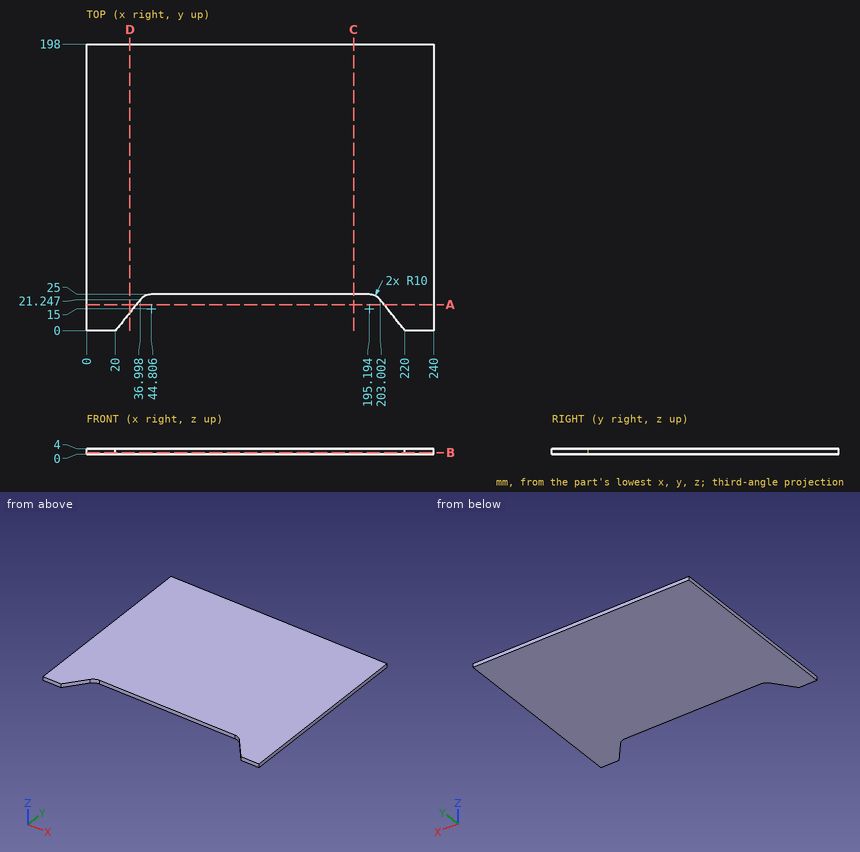
Part print with two shaded views. Sizes in mm from the minimum x, y, z corner. Round coordinates to 2 decimals unless told otherwise and drop trailing zeros. Order: outer loops, then holes, each group sorted by start corner. A loop starts at its lowest first (then second) coordinate and runs counter-clockwise, first axis right, second up. Notation, with made-up numbers: M 0.25,-0.75 L 26.25,-0.75 A16 cw 26.25,26.25 Z; hole C 84,57 d6. An arc over 180 degrees is marked long. Answer in a Markdown table with one row per item. Add a question column.
Q1. Wall check: L1, parallel to Y at x = 81.5, z = 0.35; L2, parallel to X at y = 15.5, z = 3.75; L3, parallel to Y at x = 37, z = 1.8. Give the ranges that are in metal, low to high. Write a range as from..to.
Q2. Pin check, flat tip, straight feed: pin 1 (1 mm diameter, centred on x = 51.5, z = 2, fed in from -Y). Stop position of the tip, or through.
Q3. Cut at D-D on x = 30. Give the cut face in (y, z).
Q4. Cut at C-C on x = 184.5. Give the cut face in (y, z).
Q5. Cut at A-A on y = 18. Give the cut face in (x, z).
Q6. Cut at B-B on z = 1.25. Give the cut face in (x, y), and give its area (3 significant figures).
Established:
| question | item | result |
|---|---|---|
| 1 | L1 | y = 25..198 |
| 1 | L2 | x = 0..32.4, 207.6..240 |
| 1 | L3 | y = 21.25..198 |
| 2 | pin 1 | stops at y = 25 |
| 3 | outline | M 12.5,0 L 198,0 L 198,4 L 12.5,4 Z |
| 4 | outline | M 25,0 L 198,0 L 198,4 L 25,4 Z |
| 5 | outline | M 0,0 L 34.4,0 L 34.4,4 L 0,4 Z; M 205.6,0 L 240,0 L 240,4 L 205.6,4 Z |
| 6 | outline | M 0,0 L 20,0 L 37,21.25 A10 cw 44.81,25 L 195.19,25 A10 cw 203,21.25 L 220,0 L 240,0 L 240,198 L 0,198 Z |
| 6 | area | 43,000 mm2 |
